Can you work these out from the model? Positions are in its coordinate system, mm. Coordinates: 2 decimals unless noted, no trailing zeros. Order: outer loops, then holes, each group sorted by start corner. A loop starts at its lowest first (then second) coordinate and runs counter-clockwise, first axis right, second up.
```python
from build123d import *

# Parameters (mm, degrees)
SKETCH1_W           = 25.4
SKETCH1_H           = 31.75
BOSS_EXTRUDE1_DEPTH = 3.175
SKETCH3_R           = 2.15265
CUT_EXTRUDE1_DEPTH  = 31.120694713
SKETCH4_R           = 9.525
CUT_EXTRUDE2_DEPTH  = 31.618591166


with BuildPart() as part:
    # Sketch1 → Boss-Extrude1 (new, symmetric)
    with BuildSketch(Plane(origin=(0, 0, 0), x_dir=(1, 0, 0), z_dir=(0, 1, 0))):
        with Locations((-12.7, 0)):
            Rectangle(SKETCH1_W, SKETCH1_H)
    extrude(amount=BOSS_EXTRUDE1_DEPTH, both=True)

    # Sketch3 → Cut-Extrude1 (cut, through all)
    with BuildSketch(Plane(origin=(0, 0, 0), x_dir=(0, 0, -1), z_dir=(1, 0, 0))):
        with Locations((-12.7, 0)):
            Circle(SKETCH3_R)
        with Locations((12.7, 0)):
            Circle(SKETCH3_R)
    extrude(amount=-CUT_EXTRUDE1_DEPTH, mode=Mode.SUBTRACT)

    # Sketch4 → Cut-Extrude2 (cut, through all)
    with BuildSketch(Plane(origin=(0, 3.175, 0), x_dir=(1, 0, 0), z_dir=(0, 1, 0))):
        with Locations(Location((-12.7, 0, 0), (0, 0, 270))):
            Circle(SKETCH4_R)
    extrude(amount=-CUT_EXTRUDE2_DEPTH, mode=Mode.SUBTRACT)


solid = part.part
```
1. Imagine slicing it at C-C on z = 0. Please give me the cut outline in (x, y) (3 decimals), then the cut area to 3 significant figures.
Completed:
outline: (-25.4, -3.175) - (-22.225, -3.175) - (-22.225, 3.175) - (-25.4, 3.175) - close; (-3.175, -3.175) - (0, -3.175) - (0, 3.175) - (-3.175, 3.175) - close
area: 40.3 mm2
2. Imagine slicing it at A-A on x = -12.7. Please give me the cut outline in (y, z) (3 decimals).
Completed:
outline: (-3.175, -15.875) - (3.175, -15.875) - (3.175, -9.525) - (-3.175, -9.525) - close; (-3.175, 9.525) - (3.175, 9.525) - (3.175, 15.875) - (-3.175, 15.875) - close; hole circle Ø4.305 at (0, -12.7); hole circle Ø4.305 at (0, 12.7)
3. Imagine slicing it at B-B on y = 0. Please give me the cut outline in (x, z) (3 decimals), then the cut area to 3 significant figures.
Completed:
outline: (-25.4, -15.875) - (0, -15.875) - (0, -14.853) - (-25.4, -14.853) - close; (-25.4, -10.547) - (0, -10.547) - (0, 10.547) - (-25.4, 10.547) - close; (-25.4, 14.853) - (0, 14.853) - (0, 15.875) - (-25.4, 15.875) - close; hole circle Ø19.05 at (-12.7, 0)
area: 303 mm2
4. I'm going to push a flat-ended pin straight in: pin 1 (3 mm diameter, centred on y = 1.5, z = 4, fed in from +X). Where does the tip first touch, or does it pass through?
Completed:
pin 1: stops at x = 0
5. Thinking about a two-plate mould opening in Z: for faces 1 (the cylindrical face through (-4.67, 0.04, 5.12)), 2 (the flat face through (-25.4, 0, 0)), 3 (the flat face through (-13, 0, 15.875)), which applies, pulls with the +Z half, pulls with the -Z half, needs draft (parallel to the pull), parting line crosses it, or undercut?
Completed:
face 1: undercut
face 2: needs draft
face 3: pulls with the +Z half
6. Please list where these lines run through material, in increasing order: probe 1 along Y at (x, z) = (-10.75, 12.7) (3 decimals); probe 2 along Z at (x, y) = (-14.5, -0.5) (3 decimals); probe 3 along Z at (x, y) = (-23.75, 1.5) (3 decimals).
Completed:
probe 1: y = -3.175 to -2.153, 2.153 to 3.175
probe 2: z = -15.875 to -14.794, -10.606 to -9.353, 9.353 to 10.606, 14.794 to 15.875
probe 3: z = -15.875 to -14.244, -11.156 to 11.156, 14.244 to 15.875
7. Imagine slicing it at D-D on y = 2.5. Please give me the cut outline in (x, z) (3 decimals).
Completed:
outline: (-25.4, -15.875) - (0, -15.875) - (0, 15.875) - (-25.4, 15.875) - close; hole circle Ø19.05 at (-12.7, 0)
